Source: three-view drawing plus pictorial views. Frame: mm from the lowest corner of the part. Give positions to 0.01 mm unless a question says otherwise; leave off trailing zeros. Order: outer loops, then holes, each group sorted by start corner. A loop starts at its lowest first (then second) coordinate and runs counter-clockwise, first axis right, second up.
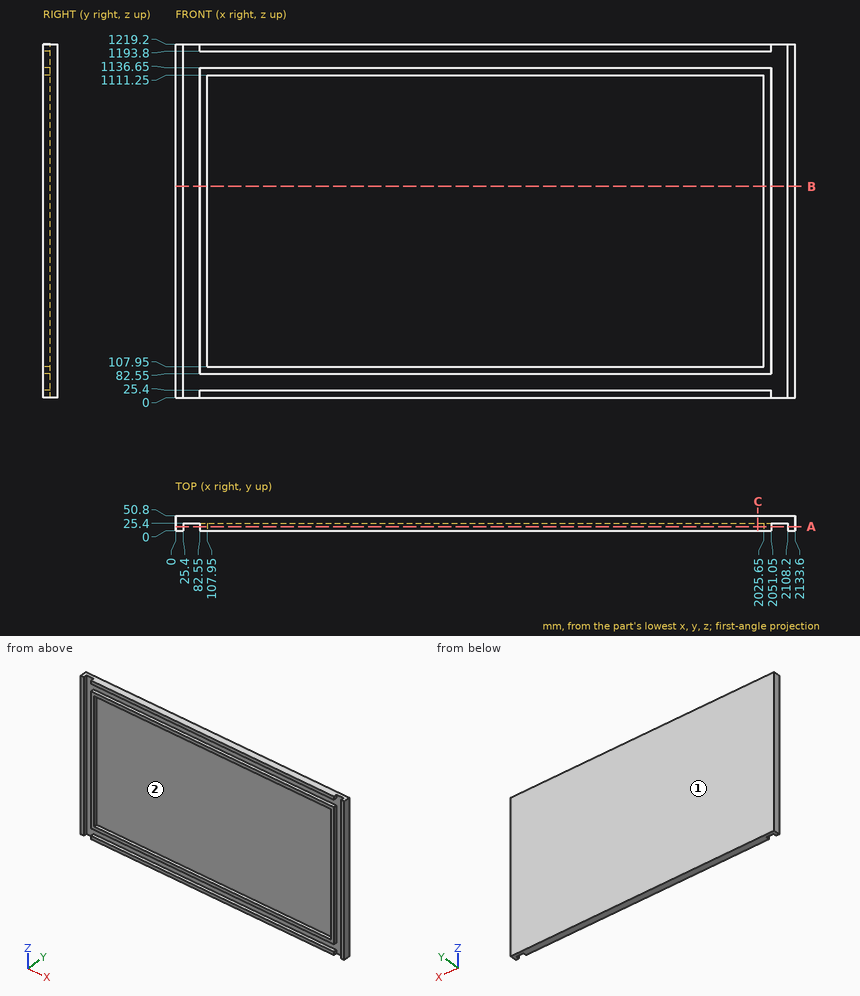
1) Section query A-A on y = 14. Output: boundary loops of the cut face in (x, z).
Checks:
outline: (0, 0) - (25.4, 0) - (25.4, 1219.2) - (0, 1219.2) - close; (82.55, 0) - (2051.05, 0) - (2051.05, 25.4) - (82.55, 25.4) - close; (82.55, 82.55) - (2051.05, 82.55) - (2051.05, 1136.65) - (82.55, 1136.65) - close; (82.55, 1193.8) - (2051.05, 1193.8) - (2051.05, 1219.2) - (82.55, 1219.2) - close; (2108.2, 0) - (2133.6, 0) - (2133.6, 1219.2) - (2108.2, 1219.2) - close; hole (107.95, 107.95) - (2025.65, 107.95) - (2025.65, 1111.25) - (107.95, 1111.25) - close
2) Section query B-B on z = 729. Output: boundary loops of the cut face in (x, y).
Checks:
outline: (0, 0) - (25.4, 0) - (25.4, 25.4) - (82.55, 25.4) - (82.55, 0) - (107.95, 0) - (107.95, 25.4) - (2025.65, 25.4) - (2025.65, 0) - (2051.05, 0) - (2051.05, 25.4) - (2108.2, 25.4) - (2108.2, 0) - (2133.6, 0) - (2133.6, 50.8) - (0, 50.8) - close
3) First-contact query: pin 1 Ø5 at (x, z) = (1557.5, 690.5) entering from -Y. Flat tip, straight axial feed; report the tip coordinate or a pass-through.
Checks:
pin 1: stops at y = 25.4
4) Section query C-C on x = 2005.5. Output: boundary loops of the cut face in (y, z), and give its area (3 significant figures).
Checks:
outline: (0, 0) - (50.8, 0) - (50.8, 1219.2) - (0, 1219.2) - (0, 1193.8) - (25.4, 1193.8) - (25.4, 1136.65) - (0, 1136.65) - (0, 1111.25) - (25.4, 1111.25) - (25.4, 107.95) - (0, 107.95) - (0, 82.55) - (25.4, 82.55) - (25.4, 25.4) - (0, 25.4) - close
area: 33,500 mm2
5) Pull-direction query (Z, two-part tool) for the marked faces 1 and 2; classes: +Z half, -Z half, draft (parallel to the pull), parting line (faces both ways), or undercut.
Checks:
face 1: draft
face 2: undercut
6) Ray query, L1, parallel to X at y = 11, z = 131; L2, parallel to Z at x = 230, y = 9.5; L3, parallel to Y at x = 1090.5, z = 485. Return the intervals inside material, ascending.
Checks:
L1: x = 0 to 25.4, 82.55 to 107.95, 2025.65 to 2051.05, 2108.2 to 2133.6
L2: z = 0 to 25.4, 82.55 to 107.95, 1111.25 to 1136.65, 1193.8 to 1219.2
L3: y = 25.4 to 50.8
